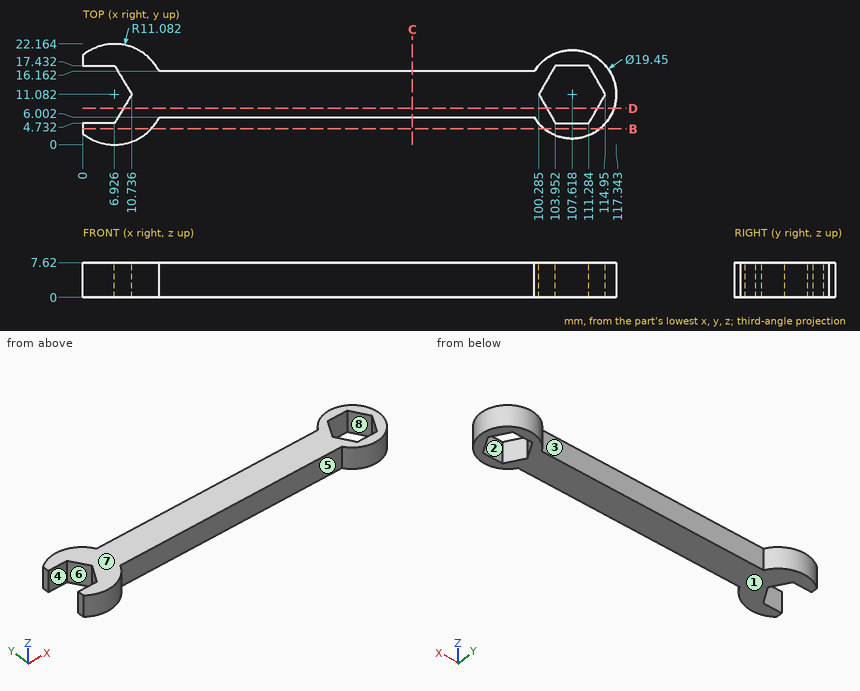
Study the drawing (mm; zero at the part's minimum x, y, z) and answer. A direction names the side the tool comes from. Coordinates: 2 decimals unless noted, no trailing zeros. Write each loop counter-clockwise with the first axis right and the second up, starting at its lowest first coordinate (ties: lowest second). Pieces come first, ordered by that corner, then holes. Notation, with made-up numbers: M 5.25,-8 L 31.25,-8 A19 cw 31.25,23 Z; hole C 43,-4 d7. An arc over 180 degrees is marked long. Write each question's results on one line, items separated by ' | '.
Item 1: Which of the six approach directions +Z, -Z, +X, -X, +Y, -Y give full straight-line access (tool end or side, diameter ignored) to the marked faces 1, 2, 3, 4 and 5?
Answer below:
face 1: -Z, +X, -X, +Y, -Y | face 2: +Z, -Z | face 3: +Z, -Z, +Y | face 4: +Z, -Z, -X | face 5: +Z, -Z, -Y
Item 2: For a pull along X with two mould halves and no side action, classify the marked faces 6, 7 and 8 as released by +X, released by -X, zero draft, split by the parting line, or undercut.
Answer below:
face 6: released by -X | face 7: zero draft | face 8: undercut
Item 3: The part is cut by section C-C on x = 72.5. Determine the outline of the cut face in (y, z).
Answer below:
outline: M 6,0 L 16.16,0 L 16.16,7.62 L 6,7.62 Z
Item 4: The part is cut by section B-B on y = 3.5. Determine the outline of the cut face in (x, z).
Answer below:
outline: M 0,0 L 15.01,0 L 15.01,7.62 L 0,7.62 Z; M 101.53,0 L 113.71,0 L 113.71,7.62 L 101.53,7.62 Z
Item 5: The part is cut by section D-D on y = 8. Determine the outline of the cut face in (x, z) (1 decimal).
Answer below:
outline: M 8.9,0 L 102.1,0 L 102.1,7.6 L 8.9,7.6 Z; M 113.2,0 L 116.8,0 L 116.8,7.6 L 113.2,7.6 Z
Item 6: Given P1, Ø3, axis at x = 99.5, y = 18.5, coming from the -Z side; P2, Ø1.5, axis at y = 19, z = 5, coming from the +X side; P3, Ø2, axis at x = 3, z = 2, coming from the -Y side; P4, Ø3.5, axis at x = 109, z = 4.5, coming from the +Y side, each flat-ended and moving along its own axis, determine where each tip first touches the part or whether it passes through.
Answer below:
P1: z = 0 | P2: x = 114.19 | P3: y = 0.39 | P4: y = 20.81
Item 7: Consider probe 1 along X at (y, z) = (5, 6.5) (1 decimal); probe 2 along X at (y, z) = (17, 3) (1 decimal); probe 3 along Y at (x, z) = (74.5, 0.5). Determine where each line is inside the solid, lowest interval first. Write a range as [from, to].
Answer below:
probe 1: [7.1, 16.2], [100, 103.8], [111.4, 115.2] | probe 2: [7.2, 16.3], [99.9, 103.7], [111.5, 115.3] | probe 3: [6, 16.16]
